The model under review builds one solid part; all positions refer to its coordinate system, in mm. A direction names the side the tool comes from. Coordinates: 2 decimals unless noted, no trailing zeros. Loops run counter-clockwise (first coordinate to the right, second up) from the corner with the lowest first, then second, coordinate; pieces in that order, holes last. Notation, with made-up numbers: (63, -3) - (93, -3) arc R8 cw to (93, 3) - close; hole circle Ø10 at (-35.75, 14). An arc over 180 degrees is marked (long way). Use a Markdown table: item, result. Add a question column.
1) Add section A-A, the plane x = 38.5. Give the boundary of the cut face in (y, z), and give its area (3 significant figures).
2) The part is to be moulded in two halves that separate along Y. For faces 4 (the cylindrical face through (12.8, -0.05, 16.07)), 5 (the cylindrical face through (51.34, -5, 42.22)), 6 (the flat face through (0, 9.525, 6)), say which applies: pulls with the +Y half, pulls with the -Y half, needs draft (parallel to the pull), parting line crosses it, or undercut.
3) To check wall thickness, follow L1, parallel to X at y = -3.25, z = -3; L2, parallel to Z at x = 10, y = -6.75; L3, parallel to X at y = -6.5, z = 9. State the ranges of each line that lie inside material, in increasing order. Write a range as [from, to].
4) Add section C-C, the plane y = 5.25. Give the boundary of the cut face in (x, z).
5) Clearance check with flat-ended pins moving along their axes: pin 1 (13 mm diameter, centred on x = 25.52, z = 25.89, fed in from +Y); pin 2 (10 mm diameter, centred on x = 15, y = 1.5, fed in from +Z); pin 3 (8.5 mm diameter, centred on y = -4, z = -6, fed in from +X). State where each tip first meets the part, or that it passes through.
6) For faces 1 (the flat face through (1, -8, 16.46)), 2 (the flat face through (15.8, 8, 8)), 3 (the flat face through (11, 0, 0)), list the 3-axis set-ups (+Z, -Z, +X, -X, +Y, -Y) from which the entire face can be reached by the end or side of a thin tool; tool diameter is ignored.
7) Add section D-D, the plane z = 8. Give the boundary of the cut face in (x, y) (3 decimals).
8) Add section B-B, the plane y = 1.5. Give the boundary of the cut face in (x, z).
```python
from build123d import *

# Parameters (mm, degrees)
F0_W     = 12.446
F0_H     = 10.407103
F1_DEPTH = 9.525
F0_R     = 4.977641
F0_R_2   = 3.889953
F0_R_3   = 2.251045
F0_R_4   = 1.016
F2_DEPTH = 6.35
F3_R     = 53.54887
F4_DEPTH = 3.683


with BuildPart() as f1:
    # F0 (on Front) → F1 (new body, symmetric)
    with BuildSketch(Plane.XZ):
        with Locations((0.093849, -5.203551)):
            Rectangle(F0_W, F0_H)
        Polygon((-15.216706, 0), (-6.129151, 0), (6.316849, 0), (15.799515, 0), (15.799515, 16.460452), (-15.216706, 16.460452), align=None)
    extrude(amount=F1_DEPTH, both=True)

    # F0 (on Front) → F2 (join, symmetric)
    with BuildSketch(Plane.XZ):
        Polygon((15.799515, 16.460452), (15.799515, 0), (61.039747, 44.118228), (61.039747, 50.637562), (50.766855, 50.637562), (-15.216706, 16.460452), align=None)
        with Locations((25.522564, 25.88735)):
            Circle(F0_R, mode=Mode.SUBTRACT)
        with Locations((38.608313, 35.421252)):
            Circle(F0_R_2, mode=Mode.SUBTRACT)
        with Locations((49.263846, 43.085761)):
            Circle(F0_R_3, mode=Mode.SUBTRACT)
        with Locations((56.371078, 47.273841)):
            Circle(F0_R_4, mode=Mode.SUBTRACT)
    extrude(amount=F2_DEPTH, both=True)

    # F3 (on Front) → F4 (cut, symmetric)
    with BuildSketch(Plane.XZ):
        with Locations((56.307051, 47.28929)):
            Circle(F3_R)
    extrude(amount=F4_DEPTH, both=True, mode=Mode.SUBTRACT)


solid = f1.part
```
From the geometry:
| question | item | result |
|---|---|---|
| 1 | outline | (-6.35, 22.14) - (-3.68, 22.14) - (-3.68, 31.53) - (-6.35, 31.53) - close; (-6.35, 39.31) - (-3.68, 39.31) - (-3.68, 44.28) - (-6.35, 44.28) - close; (3.68, 22.14) - (6.35, 22.14) - (6.35, 31.53) - (3.68, 31.53) - close; (3.68, 39.31) - (6.35, 39.31) - (6.35, 44.28) - (3.68, 44.28) - close |
| 1 | area | 76.6 mm^2 |
| 2 | face 4 | undercut |
| 2 | face 5 | needs draft |
| 2 | face 6 | pulls with the +Y half |
| 3 | L1 | x = [-6.13, 6.32] |
| 3 | L2 | z = [0, 16.46] |
| 3 | L3 | x = [-15.22, 15.8] |
| 4 | outline | (-15.22, 0) - (-6.13, 0) - (-6.13, -10.41) - (6.32, -10.41) - (6.32, 0) - (15.8, 0) - (61.04, 44.12) - (61.04, 50.64) - (50.77, 50.64) - (-15.22, 16.46) - close; hole circle Ø9.96 at (25.52, 25.89); hole circle Ø7.78 at (38.61, 35.42); hole circle Ø4.5 at (49.26, 43.09); hole circle Ø2.03 at (56.37, 47.27) |
| 5 | pin 1 | stops at y = 6.35 |
| 5 | pin 2 | stops at z = 34.44 |
| 5 | pin 3 | stops at x = 6.32 |
| 6 | face 1 | +Z, +X, -X, -Y |
| 6 | face 2 | +Z, -Z, +X, +Y |
| 6 | face 3 | -Z, +X, +Y, -Y |
| 7 | outline | (-15.217, -9.525) - (15.8, -9.525) - (15.8, -6.35) - (24.003, -6.35) - (24.003, -3.683) - (19.923, -3.683) - (19.923, 3.683) - (24.003, 3.683) - (24.003, 6.35) - (15.8, 6.35) - (15.8, 9.525) - (-15.217, 9.525) - close |
| 8 | outline | (-15.22, 0) - (-6.13, 0) - (-6.13, -10.41) - (6.32, -10.41) - (6.32, 0) - (15.8, 0) - (22.07, 6.12) arc R53.55 cw to (6.47, 27.69) - (-15.22, 16.46) - close |
